Here's how the part is built. I have some questions about the finished solid (model axes, mm). A direction names the side the tool comes from. Round coordinates to 2 decimals unless told otherwise and drop trailing zeros. Write each loop counter-clockwise with the first axis right and the second up, starting at its lowest first coordinate (ties: lowest second). Pieces come first, ordered by that corner, then holes. Notation, with made-up numbers: (-5.5, -12.5) -> (37.5, -12.5) arc R21 cw to (37.5, 17.5) -> close; hole circle Ø11 at (-28.5, 28). An arc over 180 degrees is marked (long way). Put each result on its own line as item: value. Start each with the question number.
1) I want a section at B-B, the plane y = -21.5. List the corners of the cut face in (x, z) for me.
2) If I drill on line 1 along Y through (x, z) = (0.5, 5.5); line 2 along Y through (x, z) = (100, 3.75); line 3 along Y through (x, z) = (50, 11.25), over which ranges is the centre line in solid material (lowest first)? Write a range as [from, to].
3) I want a section at C-C, the plane z = 2.25. List the corners of the cut face in (x, y) for me.
4) Which directions (+Z, -Z, +X, -X, +Y, -Y) give clear straight access to the entire face, cutting with the end or side of a thin tool? Please do faces 1 (the cylindrical face through (75.733, -70.841, 9.958)), 2 (the flat face through (53.4, -23.2, 7)), 3 (the flat face through (92.673, 4.309, 8.944)).
5) I want a section at A-A, the plane x = 72.5. List the corners of the cut face in (y, z) for me.
6) I want a section at D-D, the plane y = -64. List the corners of the cut face in (x, z) for me.
7) We'd pull the mould along X, two halves only. Please class faces 4 (the flat face through (92.673, -95.69, 8.944)), 5 (the flat face through (49, -49, 13)), 6 (the flat face through (0, 8.5, 9)), 7 (the flat face through (-19.815, -49, 5)): released by +X, released by -X, zero draft, split by the parting line, or undercut.
8) Will these pins go through, and if not, where does the flat tip stop? P1, Ø5, axis at x = 102, y = -97, coming from the +Z side; P2, Ø9, axis at x = 50, y = -21.5, coming from the -Z side.
from build123d import *

# Parameters (mm, degrees)
F0_R     = 8
F0_R_2   = 6.5
F0_R_3   = 3.5
F1_DEPTH = 13
F2_DEPTH = 13
F3_DEPTH = 7
F4_DEPTH = 13
F5_DEPTH = 5
F6_DEPTH = 5
F7_R     = 2


with BuildPart() as f1:
    # F0 (on Top) → F1 (new body)
    with BuildSketch(Plane.XY):
        with BuildLine():
            Line((99.814955, 18.5), (0.185045, 18.5))
            ThreePointArc((0.185045, 18.5), (-13.95709, 12.642136), (-19.814955, -1.5))
            Line((-19.814955, -1.5), (-19.814955, -98.5))
            ThreePointArc((-19.814955, -98.5), (-13.95709, -112.642136), (0.185045, -118.5))
            Line((0.185045, -118.5), (99.814955, -118.5))
            ThreePointArc((99.814955, -118.5), (113.95709, -112.642136), (119.814955, -98.5))
            Line((119.814955, -98.5), (119.814955, -1.5))
            ThreePointArc((119.814955, -1.5), (113.95709, 12.642136), (99.814955, 18.5))
        make_face()
        Polygon((9.814955, -100), (4.907477, -108.5), (-4.907477, -108.5), (-9.814955, -100), (-4.907477, -91.5), (4.907477, -91.5), align=None, mode=Mode.SUBTRACT)
        with Locations((27.5, -69.5)):
            Circle(F0_R, mode=Mode.SUBTRACT)
        Polygon((109.814955, -100), (104.907477, -108.5), (95.092523, -108.5), (90.185045, -100), (95.092523, -91.5), (104.907477, -91.5), align=None, mode=Mode.SUBTRACT)
        with Locations((72.5, -69.5)):
            Circle(F0_R, mode=Mode.SUBTRACT)
        with Locations((50, -21.5)):
            Circle(F0_R, mode=Mode.SUBTRACT)
        Polygon((9.814955, 0), (4.907477, -8.5), (-4.907477, -8.5), (-9.814955, 0), (-4.907477, 8.5), (4.907477, 8.5), align=None, mode=Mode.SUBTRACT)
        Polygon((109.814955, 0), (104.907477, -8.5), (95.092523, -8.5), (90.185045, 0), (95.092523, 8.5), (104.907477, 8.5), align=None, mode=Mode.SUBTRACT)
        Polygon((-4.907477, -8.5), (4.907477, -8.5), (9.814955, 0), (4.907477, 8.5), (-4.907477, 8.5), (-9.814955, 0), align=None)
        Circle(F0_R_2, mode=Mode.SUBTRACT)
        with Locations((50, -21.5)):
            Circle(F0_R)
        with Locations((50, -21.5)):
            Circle(F0_R_3, mode=Mode.SUBTRACT)
        with Locations((50, -21.5)):
            Circle(F0_R_3)
        Polygon((95.092523, -8.5), (104.907477, -8.5), (109.814955, 0), (104.907477, 8.5), (95.092523, 8.5), (90.185045, 0), align=None)
        with Locations((100, 0)):
            Circle(F0_R_2, mode=Mode.SUBTRACT)
        with Locations((72.5, -69.5)):
            Circle(F0_R)
        with Locations((72.5, -69.5)):
            Circle(F0_R_3, mode=Mode.SUBTRACT)
        with Locations((72.5, -69.5)):
            Circle(F0_R_3)
        with Locations((27.5, -69.5)):
            Circle(F0_R)
        with Locations((27.5, -69.5)):
            Circle(F0_R_3, mode=Mode.SUBTRACT)
        with Locations((27.5, -69.5)):
            Circle(F0_R_3)
        Polygon((-4.907477, -108.5), (4.907477, -108.5), (9.814955, -100), (4.907477, -91.5), (-4.907477, -91.5), (-9.814955, -100), align=None)
        with Locations((0, -100)):
            Circle(F0_R_2, mode=Mode.SUBTRACT)
        Polygon((95.092523, -108.5), (104.907477, -108.5), (109.814955, -100), (104.907477, -91.5), (95.092523, -91.5), (90.185045, -100), align=None)
        with Locations((100, -100)):
            Circle(F0_R_2, mode=Mode.SUBTRACT)
    extrude(amount=F1_DEPTH)

    # F0 (on Top) → F2 (cut, through all)
    with BuildSketch(Plane.XY):
        Polygon((-4.907477, -8.5), (4.907477, -8.5), (9.814955, 0), (4.907477, 8.5), (-4.907477, 8.5), (-9.814955, 0), align=None)
        Circle(F0_R_2, mode=Mode.SUBTRACT)
        Polygon((95.092523, -108.5), (104.907477, -108.5), (109.814955, -100), (104.907477, -91.5), (95.092523, -91.5), (90.185045, -100), align=None)
        with Locations((100, -100)):
            Circle(F0_R_2, mode=Mode.SUBTRACT)
        Polygon((-4.907477, -108.5), (4.907477, -108.5), (9.814955, -100), (4.907477, -91.5), (-4.907477, -91.5), (-9.814955, -100), align=None)
        with Locations((0, -100)):
            Circle(F0_R_2, mode=Mode.SUBTRACT)
        Polygon((95.092523, -8.5), (104.907477, -8.5), (109.814955, 0), (104.907477, 8.5), (95.092523, 8.5), (90.185045, 0), align=None)
        with Locations((100, 0)):
            Circle(F0_R_2, mode=Mode.SUBTRACT)
    extrude(amount=F2_DEPTH, mode=Mode.SUBTRACT)

    # F0 (on Top) → F3 (cut)
    with BuildSketch(Plane.XY):
        with Locations((72.5, -69.5)):
            Circle(F0_R)
        with Locations((72.5, -69.5)):
            Circle(F0_R_3, mode=Mode.SUBTRACT)
        with Locations((27.5, -69.5)):
            Circle(F0_R)
        with Locations((27.5, -69.5)):
            Circle(F0_R_3, mode=Mode.SUBTRACT)
        with Locations((50, -21.5)):
            Circle(F0_R)
        with Locations((50, -21.5)):
            Circle(F0_R_3, mode=Mode.SUBTRACT)
    extrude(amount=F3_DEPTH, mode=Mode.SUBTRACT)

    # F0 (on Top) → F4 (cut, through all)
    with BuildSketch(Plane.XY):
        with Locations((27.5, -69.5)):
            Circle(F0_R_3)
        with Locations((72.5, -69.5)):
            Circle(F0_R_3)
        with Locations((50, -21.5)):
            Circle(F0_R_3)
    extrude(amount=F4_DEPTH, mode=Mode.SUBTRACT)

    # F0 (on Top) → F5 (join)
    with BuildSketch(Plane.XY):
        Polygon((-4.907477, -8.5), (4.907477, -8.5), (9.814955, 0), (4.907477, 8.5), (-4.907477, 8.5), (-9.814955, 0), align=None)
        Circle(F0_R_2, mode=Mode.SUBTRACT)
        Polygon((95.092523, -8.5), (104.907477, -8.5), (109.814955, 0), (104.907477, 8.5), (95.092523, 8.5), (90.185045, 0), align=None)
        with Locations((100, 0)):
            Circle(F0_R_2, mode=Mode.SUBTRACT)
        Polygon((95.092523, -108.5), (104.907477, -108.5), (109.814955, -100), (104.907477, -91.5), (95.092523, -91.5), (90.185045, -100), align=None)
        with Locations((100, -100)):
            Circle(F0_R_2, mode=Mode.SUBTRACT)
        Polygon((-4.907477, -108.5), (4.907477, -108.5), (9.814955, -100), (4.907477, -91.5), (-4.907477, -91.5), (-9.814955, -100), align=None)
        with Locations((0, -100)):
            Circle(F0_R_2, mode=Mode.SUBTRACT)
    extrude(amount=F5_DEPTH)

    # F0 (on Top) → F6 (cut, through all)
    with BuildSketch(Plane.XY):
        Circle(F0_R_2)
        with Locations((100, 0)):
            Circle(F0_R_2)
        with Locations((100, -100)):
            Circle(F0_R_2)
        with Locations((0, -100)):
            Circle(F0_R_2)
    extrude(amount=F6_DEPTH, mode=Mode.SUBTRACT)

    # F7
    f7_edges = [f1.edges().sort_by_distance(p)[0] for p in [
        (119.814955, -50, 13),
    ]]
    fillet(f7_edges, radius=F7_R)


solid = f1.part
Findings:
1. outline: (-19.81, 0) -> (42, 0) -> (42, 7) -> (46.5, 7) -> (46.5, 13) -> (-17.81, 13) arc R2 ccw to (-19.81, 11) -> close; (53.5, 7) -> (58, 7) -> (58, 0) -> (119.81, 0) -> (119.81, 11) arc R2 ccw to (117.81, 13) -> (53.5, 13) -> close
2. line 1: y = [-118.5, -108.5], [-91.5, -8.5], [8.5, 18.5]
2. line 2: y = [-118.5, -106.5], [-93.5, -6.5], [6.5, 18.5]
2. line 3: y = [-118.48, -25], [-18, 18.48]
3. outline: (-19.81, -98.5) arc R20 ccw to (0.19, -118.5) -> (99.81, -118.5) arc R20 ccw to (119.81, -98.5) -> (119.81, -1.5) arc R20 ccw to (99.81, 18.5) -> (0.19, 18.5) arc R20 ccw to (-19.81, -1.5) -> close; hole circle Ø13 at (0, -100); hole circle Ø13 at (0, 0); hole circle Ø16 at (27.5, -69.5); hole circle Ø16 at (50, -21.5); hole circle Ø16 at (72.5, -69.5); hole circle Ø13 at (100, -100); hole circle Ø13 at (100, 0)
4. face 1: +Z, -Z
4. face 2: -Z
4. face 3: +Z
5. outline: (-118.5, 0) -> (-77.5, 0) -> (-77.5, 7) -> (-73, 7) -> (-73, 13) -> (-116.5, 13) arc R2 ccw to (-118.5, 11) -> close; (-66, 7) -> (-61.5, 7) -> (-61.5, 0) -> (18.5, 0) -> (18.5, 11) arc R2 ccw to (16.5, 13) -> (-66, 13) -> close
6. outline: (-19.81, 0) -> (21.69, 0) -> (21.69, 7) -> (33.31, 7) -> (33.31, 0) -> (66.69, 0) -> (66.69, 7) -> (78.31, 7) -> (78.31, 0) -> (119.81, 0) -> (119.81, 11) arc R2 ccw to (117.81, 13) -> (-17.81, 13) arc R2 ccw to (-19.81, 11) -> close
7. face 4: undercut
7. face 5: zero draft
7. face 6: undercut
7. face 7: released by -X
8. P1: passes through
8. P2: stops at z = 7
